Work out the finished part from the listing and answer in its coordinate system (mm). A direction names the side the tool comes from. Give positions to 0.01 mm unless a question says otherwise; leave off trailing zeros. Loops run counter-clockwise (first coordinate to the right, second up) from the corner with the lowest first, then second, coordinate; pieces in that order, holes last.
from build123d import *

# Parameters (mm, degrees)
BOSS_EXTRUDE1_DEPTH = 25.4
CUT_EXTRUDE1_REACH  = 369.204
SKETCH2_R           = 12.7
SKETCH3_R           = 9.525
CUT_EXTRUDE2_DEPTH  = 50.8
SKETCH4_R           = 6.35
BOSS_EXTRUDE2_DEPTH = 68.58
CUT_EXTRUDE3_DEPTH  = 19.05


with BuildPart() as part:
    # Sketch1 → Boss-Extrude1 (new, symmetric)
    with BuildSketch(Plane.XY):
        Polygon((0, 0), (0, 203.2), (50.8, 203.2), (50.8, 50.8), (254, 50.8), (254, 165.1), (304.8, 165.1), (304.8, 0), align=None)
    extrude(amount=BOSS_EXTRUDE1_DEPTH, both=True)

    # Sketch2 → Cut-Extrude1 (cut, up to next)
    with BuildSketch(Plane.ZY, mode=Mode.PRIVATE) as cut_extrude1_sk1:
        with Locations((0, 177.8)):
            Circle(SKETCH2_R)
    cut_extrude1_tool1 = extrude(cut_extrude1_sk1.sketch, amount=-CUT_EXTRUDE1_REACH, mode=Mode.PRIVATE) & part.part
    add(cut_extrude1_tool1.solids().sort_by_distance((0, 177.8, 0))[0], mode=Mode.SUBTRACT)

    # Sketch3 → Cut-Extrude2 (cut)
    with BuildSketch(Plane.ZY):
        with Locations((0, 63.5)):
            Circle(SKETCH3_R)
    extrude(amount=-CUT_EXTRUDE2_DEPTH, mode=Mode.SUBTRACT)

    # Sketch4 → Boss-Extrude2 (add)
    with BuildSketch(Plane.XY.offset(25.4)):
        with Locations(Location((144.449989541, 24.404106045, 0), (0, 0, 180))):
            Circle(SKETCH4_R)
    extrude(amount=BOSS_EXTRUDE2_DEPTH)

    # Sketch5 → Cut-Extrude3 (cut)
    with BuildSketch(Plane(origin=(0, 50.8, 0), x_dir=(1, 0, 0), z_dir=(0, 1, 0))):
        with BuildLine():
            ThreePointArc((227.02055062, -6.025839331), (153.726793571, 17.638579798), (80.433036521, -6.025839331))
            ThreePointArc((80.433036521, -6.025839331), (78.995330638, -14.890262707), (87.859754015, -16.32796859))
            ThreePointArc((87.859754015, -16.32796859), (153.726793571, 4.938579798), (219.593833127, -16.32796859))
            ThreePointArc((219.593833127, -16.32796859), (228.458256503, -14.890262707), (227.02055062, -6.025839331))
        make_face()
    extrude(amount=-CUT_EXTRUDE3_DEPTH, mode=Mode.SUBTRACT)


solid = part.part
Item 1: Find section D-D, the plane x = 145.5. Write down the section's boundary in (y, z).
Item 2: For faces 1 (the face through (154.823, 41.408, -17.634)), 2 (the face through (279, 165.1, 0)), 3 (the face through (254, 107, 0)), 4 (the face through (149.49, 28.27, 59.21)), determine the directions among +Z, -Z, +X, -X, +Y, -Y from which every point of the face is accessible in a straight line to the end or side of a thin tool.
Item 3: Consider line 1 (Y direction, x = 11.5, z = 0) (3 decimals); line 2 (X direction, y = 161.5, z = -15.5); line 3 (Y direction, x = 35, z = 3). Determine where each line is inside the solid, lowest interval first.
Item 4: Determine the mould class of faces 5 (the face through (25.044, 188.509, 6.827)), 6 (the face through (153, 31.75, -8)), 7 (the face through (152.742, 41.408, -4.934)) for opening direction Y: released by +Y, released by -Y, zero draft, split by the parting line, or undercut.
Item 5: Find section A-A, the plane y = 63.5. Write down the section's boundary in (x, z) (3 decimals), plus the area to 3 significant figures.
Item 6: Find section B-B, the plane y = 177.8. Write down the section's boundary in (x, z), plus the area to 3 significant figures.
Item 7: Find section C-C, the plane z = 0. Write down the section's boundary in (x, y) (3 decimals), plus the area to 3 significant figures.
Item 8: Flat-ended cylindrical pins translate along their axes: pin 1 Ø6 at (y, z) = (32, 59) entering from -X; pin 2 Ø17.5 at (x, z) = (169, -5) entering from +Y. Find the tip coordinate at first contact, or state that the pin passes through.
Ans:
1. outline: (0, -25.4) - (50.8, -25.4) - (50.8, -17.37) - (31.75, -17.37) - (31.75, -4.64) - (50.8, -4.64) - (50.8, 25.4) - (30.67, 25.4) - (30.67, 93.98) - (18.14, 93.98) - (18.14, 25.4) - (0, 25.4) - close
2. face 1: +Y
2. face 2: +Z, -Z, +X, +Y
2. face 3: +Z, -Z, +Y
2. face 4: +Z
3. line 1: y = 0 to 53.975, 73.025 to 165.1, 190.5 to 203.2
3. line 2: x = 0 to 50.8, 254 to 304.8
3. line 3: y = 0 to 54.46, 72.54 to 165.46, 190.14 to 203.2
4. face 5: undercut
4. face 6: released by +Y
4. face 7: zero draft
5. outline: (0, -25.4) - (50.8, -25.4) - (50.8, -9.525) - (0, -9.525) - close; (0, 9.525) - (50.8, 9.525) - (50.8, 25.4) - (0, 25.4) - close; (254, -25.4) - (304.8, -25.4) - (304.8, 25.4) - (254, 25.4) - close
5. area: 4,190 mm2
6. outline: (0, -25.4) - (50.8, -25.4) - (50.8, -12.7) - (0, -12.7) - close; (0, 12.7) - (50.8, 12.7) - (50.8, 25.4) - (0, 25.4) - close
6. area: 1,290 mm2
7. outline: (0, 0) - (304.8, 0) - (304.8, 165.1) - (254, 165.1) - (254, 50.8) - (217.839, 50.8) - (217.839, 31.75) - (186.714, 31.75) - (186.714, 50.8) - (120.74, 50.8) - (120.74, 31.75) - (89.615, 31.75) - (89.615, 50.8) - (50.8, 50.8) - (50.8, 53.975) - (0, 53.975) - close; (0, 73.025) - (50.8, 73.025) - (50.8, 165.1) - (0, 165.1) - close; (0, 190.5) - (50.8, 190.5) - (50.8, 203.2) - (0, 203.2) - close
7. area: 25,600 mm2
8. pin 1: stops at x = 140.07
8. pin 2: stops at y = 50.8
